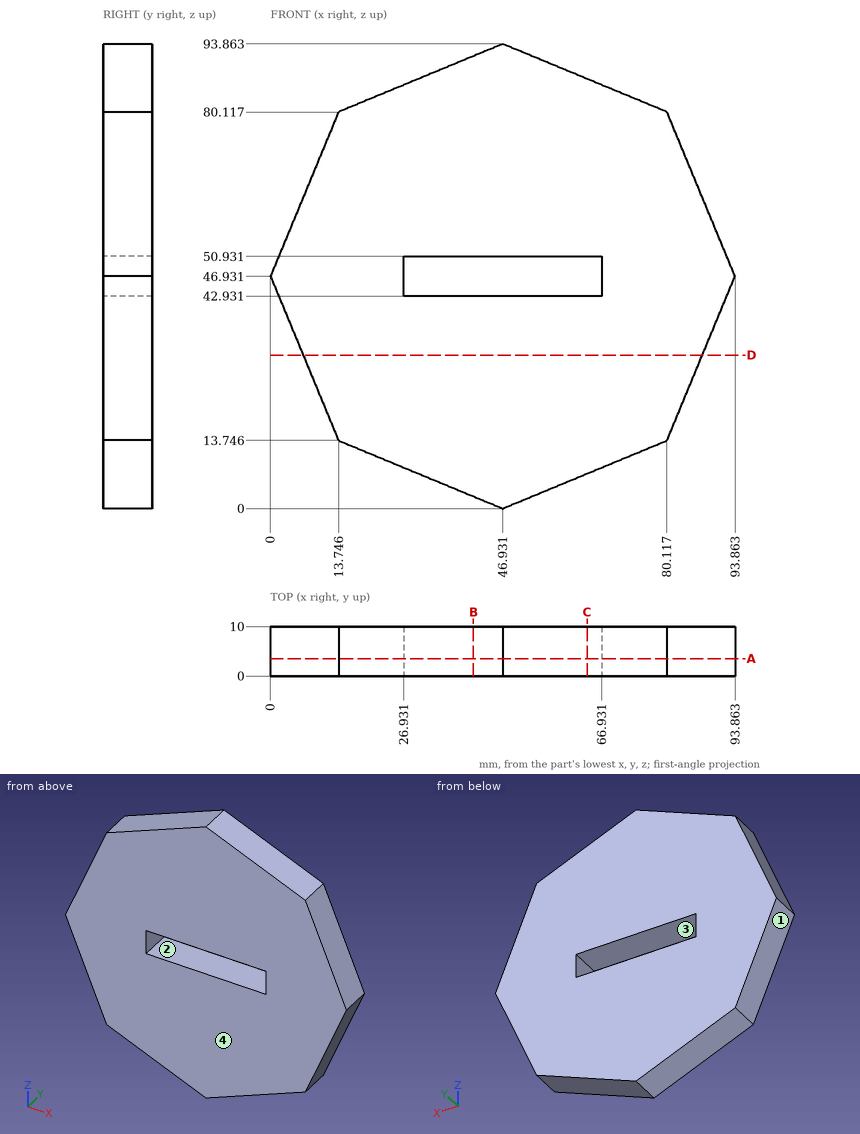
Print and shaded views of the part. All mm, measured from the part's lowest x, y and z. Coordinates: 2 decimals unless noted, no trailing zeros. Loops run counter-clockwise (first coordinate to the right, second up) from the corner with the lowest first, then second, coordinate; pieces in that order, holes last. Notation, with made-up numbers: M -24.5,78.25 L 2.5,78.25 A20 ccw 2.5,96.25 Z; hole C 64,69 d11. An arc over 180 degrees is marked long. Use a Markdown table: item, result. Add a question column.
Q1. Cut at B-B (x = 41). Write the cut outline in (y, z).
Q2. Cut at C-C (x = 64). Write the cut outline in (y, z).
Q3. Probe L1, parallel to Z at x = 59.5, y = 2.75 (1 decimal); L2, parallel to X at y = 5.75, z = 43 (1 decimal); L3, parallel to Z at x = 35, y = 8.5. List the from-to ranges inside material, lowest first.
Q4. Mould opens along X. For the marked faces 1, 2, 3 and 4 say: +X half, -X half, draft (parallel to the pull), parting line (faces both ways), or undercut.
Q5. Cut at A-A (y = 3.5). Write the cut outline in (x, z), and give its area (3 significant figures).
Q6. Cut at D-D (z = 31). Write the cut outline in (x, y).
Q7. Pin check, flat tips, straight feed: P1, Ø1.5, axis at y = 1, z = 79.5, coming from the +X side; P2, Ø5, axis at y = 9, z = 24.5, coming from the +X side; P3, Ø2.5, axis at y = 4.5, z = 49, coming from the +X side. Stop position of each tip, or through.
Worked out:
| question | item | result |
|---|---|---|
| 1 | outline | M 0,2.46 L 10,2.46 L 10,42.93 L 0,42.93 Z; M 0,50.93 L 10,50.93 L 10,91.41 L 0,91.41 Z |
| 2 | outline | M 0,7.07 L 10,7.07 L 10,42.93 L 0,42.93 Z; M 0,50.93 L 10,50.93 L 10,86.79 L 0,86.79 Z |
| 3 | L1 | z = 5.2 to 42.9, 50.9 to 88.7 |
| 3 | L2 | x = 1.6 to 26.9, 66.9 to 92.2 |
| 3 | L3 | z = 4.94 to 42.93, 50.93 to 88.92 |
| 4 | face 1 | -X half |
| 4 | face 2 | undercut |
| 4 | face 3 | undercut |
| 4 | face 4 | draft |
| 5 | outline | M 0,46.93 L 13.75,13.75 L 46.93,0 L 80.12,13.75 L 93.86,46.93 L 80.12,80.12 L 46.93,93.86 L 13.75,80.12 Z; hole M 26.93,42.93 L 66.93,42.93 L 66.93,50.93 L 26.93,50.93 Z |
| 5 | area | 5,910 mm2 |
| 6 | outline | M 6.6,0 L 87.26,0 L 87.26,10 L 6.6,10 Z |
| 7 | P1 | stops at x = 80.68 |
| 7 | P2 | stops at x = 85.61 |
| 7 | P3 | stops at x = 93.52 |
